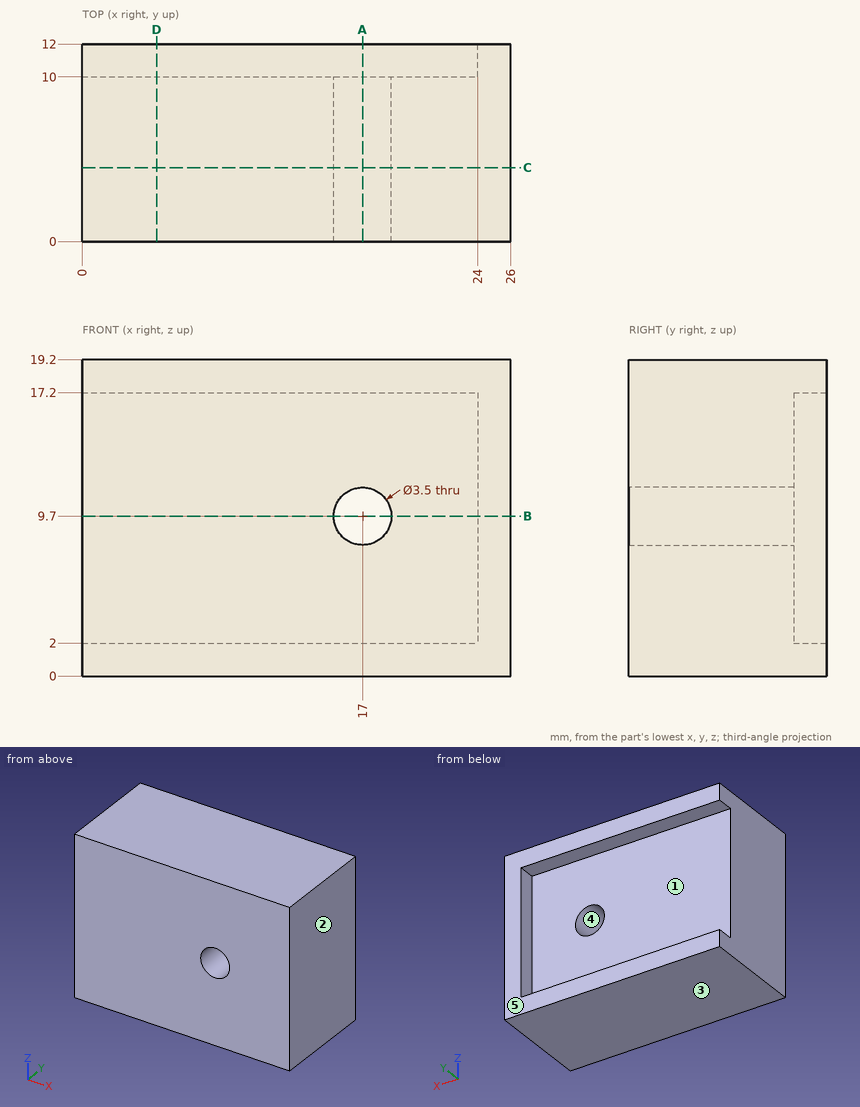
Source: three-view drawing plus pictorial views. Frame: mm from the lowest corner of the part. A direction names the side the tool comes from. Coordinates: 2 decimals unless noted, no trailing zeros. Write each loop counter-clockwise with the first axis right and the second up, starting at its lowest first coordinate (ties: lowest second). Pieces come first, ordered by that corner, then holes. Notation, with made-up numbers: (-11, 4.5) -> (-2, 4.5) arc R26 ccw to (-2, 32.5) -> close; hole circle Ø6 at (-2.5, -5). An arc over 180 degrees is marked (long way). Answer as a JSON object with one key per item and string values.
1. Section C-C on y = 4.5. Return the cut outline in (x, z), then the cut area to 3 significant figures.
Result set:
{"outline": "(0, 0) -> (26, 0) -> (26, 19.2) -> (0, 19.2) -> close; hole circle Ø3.5 at (17, 9.7)", "area": "490 mm2"}
2. Section B-B on z = 9.7. Return the cut outline in (x, y), then the cut area to 3 significant figures.
Result set:
{"outline": "(0, 0) -> (15.25, 0) -> (15.25, 10) -> (0, 10) -> close; (18.75, 0) -> (26, 0) -> (26, 12) -> (24, 12) -> (24, 10) -> (18.75, 10) -> close", "area": "229 mm2"}
3. Access query for the marked faces 1 and 2. Directions: +Z, -Z, +X, -X, +Y, -Y. A direction counts if a zero-diameter tool reaches every point of the face in a straight line with its end or side. Return the directions, or none.
Result set:
{"face 1": "-X, +Y", "face 2": "+Z, -Z, +X, +Y, -Y"}
4. Material intervals for line 1 (X direction, y = 6.25, z = 9.7); line 2 (Z direction, x = 14.25, y = 11); line 3 (X direction, y = 11.75, z = 13.5), sorted ascending. Write a range as from..to.
Result set:
{"line 1": "x = 0..15.25, 18.75..26", "line 2": "z = 0..2, 17.2..19.2", "line 3": "x = 24..26"}
5. Mould query, pull axis Z, two halves, no side actions, for the marked faces 3, 4 and 5. Classes: released by +Z, released by -Z, zero draft, split by the parting line, or undercut.
Result set:
{"face 3": "released by -Z", "face 4": "undercut", "face 5": "zero draft"}
6. First-contact query: P1, Ø1, axis at x = 6.5, y = 2.5, coming from the -Z side; P2, Ø4.5, axis at x = 14, z = 6.5, coming from the +Y side. Flat tips, straight axial feed; report the tip coordinate or a pass-through.
Result set:
{"P1": "stops at z = 0", "P2": "stops at y = 10"}
7. Section D-D on x = 4.5. Return the cut outline in (y, z), then the cut area to 3 significant figures.
Result set:
{"outline": "(0, 0) -> (12, 0) -> (12, 2) -> (10, 2) -> (10, 17.2) -> (12, 17.2) -> (12, 19.2) -> (0, 19.2) -> close", "area": "200 mm2"}
8. Section A-A on x = 17. Return the cut outline in (y, z), then the cut area to 3 significant figures.
Result set:
{"outline": "(0, 0) -> (12, 0) -> (12, 2) -> (10, 2) -> (10, 7.95) -> (0, 7.95) -> close; (0, 11.45) -> (10, 11.45) -> (10, 17.2) -> (12, 17.2) -> (12, 19.2) -> (0, 19.2) -> close", "area": "165 mm2"}
